Read the model definition and answer for the solid it produces. Units are mm, in the model's axes. Coordinates: 2 decimals unless noted, no trailing zeros. Order: outer loops, then holes, each group sorted by start corner. A loop starts at its lowest first (then second) coordinate and runs counter-clockwise, first axis right, second up. Notation, with made-up numbers: M 24,4.5 L 71,4.5 A20 cw 71,37.5 Z; hole C 47.25,73 d11. An arc over 180 degrees is marked long. Put each result on its own line as item: value.
from build123d import *

# Parameters (mm, degrees)
F0_R     = 150
F1_DEPTH = 20
F3_DEPTH = 20.001
F4_R     = 5
F5_DEPTH = 20.001


with BuildPart() as f1:
    # F0 (on Top) → F1 (new body)
    with BuildSketch(Plane.XY):
        Circle(F0_R)
    extrude(amount=F1_DEPTH)

    # F2 (on face) → F3 (cut, through all)
    with BuildSketch(Plane.XY.offset(20)):
        with BuildLine():
            ThreePointArc((-2.499860907, 118.473628692), (0, 118.5), (2.499860907, 118.473628692))
            ThreePointArc((2.499860907, 118.473628692), (2.4999652265, 118.4868141626), (2.5, 118.5))
            ThreePointArc((2.5, 118.5), (-0.0131858374, 120.9999652265), (-2.499860907, 118.473628692))
        make_face()
        with BuildLine():
            ThreePointArc((-2.499860907, 118.473628692), (0, 116), (2.499860907, 118.473628692))
            ThreePointArc((2.499860907, 118.473628692), (0, 118.5), (-2.499860907, 118.473628692))
        make_face()
        with BuildLine():
            ThreePointArc((-118.473628692, -2.499860907), (-118.5, 0), (-118.473628692, 2.499860907))
            ThreePointArc((-118.473628692, 2.499860907), (-121, 0), (-118.473628692, -2.499860907))
        make_face()
        with BuildLine():
            ThreePointArc((-116, 0), (-116.7229338406, 1.7584185693), (-118.473628692, 2.499860907))
            ThreePointArc((-118.473628692, 2.499860907), (-118.5, 0), (-118.473628692, -2.499860907))
            ThreePointArc((-118.473628692, -2.499860907), (-116.7229338406, -1.7584185693), (-116, 0))
        make_face()
        with BuildLine():
            ThreePointArc((118.473628692, -2.499860907), (118.4934069896, -1.25), (118.5, 0))
            ThreePointArc((118.5, 0), (118.4934069896, 1.25), (118.473628692, 2.499860907))
            ThreePointArc((118.473628692, 2.499860907), (116, 0), (118.473628692, -2.499860907))
        make_face()
        with BuildLine():
            ThreePointArc((118.473628692, 2.499860907), (118.4934069896, 1.25), (118.5, 0))
            ThreePointArc((118.5, 0), (118.4934069896, -1.25), (118.473628692, -2.499860907))
            ThreePointArc((118.473628692, -2.499860907), (120.2584185693, -1.7770661594), (121, 0))
            ThreePointArc((121, 0), (120.2584185693, 1.7770661594), (118.473628692, 2.499860907))
        make_face()
        with BuildLine():
            ThreePointArc((-2.499860907, -118.473628692), (0, -118.5), (2.499860907, -118.473628692))
            ThreePointArc((2.499860907, -118.473628692), (0, -116), (-2.499860907, -118.473628692))
        make_face()
        with BuildLine():
            ThreePointArc((2.5, -118.5), (2.4999652265, -118.4868141626), (2.499860907, -118.473628692))
            ThreePointArc((2.499860907, -118.473628692), (0, -118.5), (-2.499860907, -118.473628692))
            ThreePointArc((-2.499860907, -118.473628692), (-0.0131858374, -120.9999652265), (2.5, -118.5))
        make_face()
    extrude(amount=-F3_DEPTH, mode=Mode.SUBTRACT)

    # F4 (on face) → F5 (cut, through all)
    with BuildSketch(Plane.XY.offset(20)):
        Circle(F4_R)
        with Locations((30, 0)):
            Circle(F4_R)
        with Locations((60, 0)):
            Circle(F4_R)
        with Locations((-30, 0)):
            Circle(F4_R)
        with Locations((-60, 0)):
            Circle(F4_R)
    extrude(amount=-F5_DEPTH, mode=Mode.SUBTRACT)


solid = f1.part
Q1. Find section A-A on z = 16.25. Give the number of separate pieces and of enclosed holes in the cut face, plus the area to 3 significant figures.
Answers below:
separate pieces: 1
enclosed holes: 9
area: 70,200 mm^2
Q2. Consider line 1 along Y through (x, z) = (0, 13.25); line 2 along Y through (x, z) = (-60, 4); line 3 along Y through (x, z) = (30, 9.5). Determine where each line is inside the solid, lowest interval first.
Answers below:
line 1: y = -150 to -121, -116 to -5, 5 to 116, 121 to 150
line 2: y = -137.48 to -5, 5 to 137.48
line 3: y = -146.97 to -5, 5 to 146.97
Q3. Find section C-C on x = -60. Write down the section's boundary in (y, z), plus the area to 3 significant figures.
Answers below:
outline: M -137.48,0 L -5,0 L -5,20 L -137.48,20 Z; M 5,0 L 137.48,0 L 137.48,20 L 5,20 Z
area: 5,300 mm^2
Q4. Find section D-D on y = -91. Write down the section's boundary in (x, z), plus the area to 3 significant figures.
Answers below:
outline: M -119.24,0 L 119.24,0 L 119.24,20 L -119.24,20 Z
area: 4,770 mm^2
Q5. Given pin 1 (16 mm diameter, centred on x = 60, y = 0, fed in from +Z); pin 2 (6 mm diameter, centred on y = -53, z = 18, fed in from +X); pin 3 (4 mm diameter, centred on x = -57, z = 13, fed in from +Y); pin 4 (4 mm diameter, centred on x = -114.5, z = 4.5, fed in from -Y), each flat-ended and moving along its own axis, determine where each tip first touches the part or whether it passes through.
Answers below:
pin 1: stops at z = 20
pin 2: stops at x = 141.42
pin 3: stops at y = 139.55
pin 4: stops at y = -99.22
Q6. Find section B-B on x = 30. Write down the section's boundary in (y, z), plus the area to 3 significant figures.
Answers below:
outline: M -146.97,0 L -5,0 L -5,20 L -146.97,20 Z; M 5,0 L 146.97,0 L 146.97,20 L 5,20 Z
area: 5,680 mm^2
Q7. For a pull along X with two mould halves and no side action, classify faces 1 (the face through (-19.527, 148.724, 9.86)), 2 (the face through (-35, 0, 10)), 3 (the face through (-2, -31, 0)), 4 (the face through (25, 0, 10)) as +X half, -X half, draft (parallel to the pull), parting line (faces both ways), or undercut.
Answers below:
face 1: parting line
face 2: undercut
face 3: draft
face 4: undercut
